Check sheet for the modelled part. Datum: model origin and axes. Units: mm. Give positions to 0.01 mm unless a question says otherwise; leave off trailing zeros. Order: outer loops, then holes, each group sorted by start corner. A loop starts at its lowest first (then second) coordinate and runs counter-clockwise, first axis right, second up.
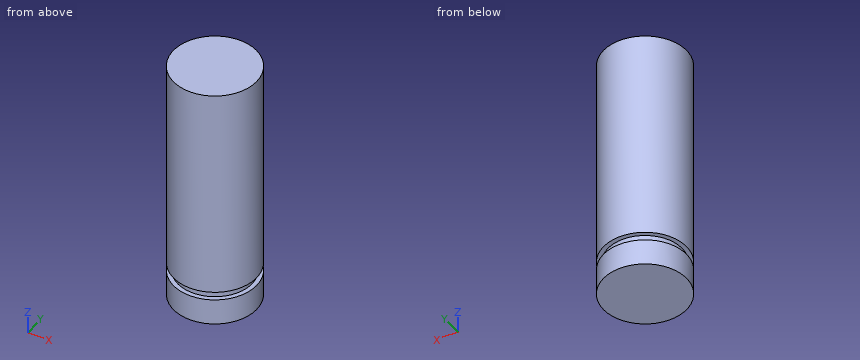
from build123d import *

# Parameters (mm, degrees)
SKETCH1_R           = 3.025
BOSS_EXTRUDE1_DEPTH = 18


with BuildPart() as part:
    # Sketch1 → Boss-Extrude1 (new body)
    with BuildSketch(Plane.XY):
        Circle(SKETCH1_R)
    extrude(amount=BOSS_EXTRUDE1_DEPTH)

    # Sketch3 → Groove for ANSI B27.7 - 3BM1-8, Basic Internal Retaining Ring1 (revolve, cut)
    with BuildSketch(Plane(origin=(0, 0, 18), x_dir=(0, 1, 0), z_dir=(-1, 0, 0)), mode=Mode.PRIVATE) as groove_for_ansi_b27_7_3bm1_8_basic_in_sk:
        with BuildLine():
            Line((4.1, 15.5), (2.7, 15.5))
            Line((2.7, 15.5), (2.7, 16.1))
            Line((2.7, 16.1), (4.1, 16.1))
            ThreePointArc((4.1, 16.1), (4.170710678, 16.070710678), (4.2, 16))
            Line((4.2, 16), (4.2, 15.6))
            ThreePointArc((4.2, 15.6), (4.170710678, 15.529289322), (4.1, 15.5))
        make_face()
    revolve(groove_for_ansi_b27_7_3bm1_8_basic_in_sk.sketch.rotate(Axis((0, 0, 68), (0, 0, -1)), 270), axis=Axis((0, 0, 68), (0, 0, -1)), mode=Mode.SUBTRACT)


solid = part.part
1) Depth check by flat-ended pin: pin 1 Ø1 at (x, z) = (2, 10.5) entering from -Y. Enter the tip coordinate at first touch or a pass-through.
Recorded:
pin 1: stops at y = -2.63
2) Section check B-B, the plane z = 10. Record the cut outline in (x, y) (3 decimals), then the cut area to 3 significant figures.
Recorded:
outline: circle Ø6.05 at (0, 0)
area: 28.7 mm2
3) Section check C-C, the plane y = -1. Record the cut outline in (x, z), then the cut area to 3 significant figures.
Recorded:
outline: (-2.85, 0) - (2.85, 0) - (2.85, 1.9) - (2.51, 1.9) - (2.51, 2.5) - (2.85, 2.5) - (2.85, 18) - (-2.85, 18) - (-2.85, 2.5) - (-2.51, 2.5) - (-2.51, 1.9) - (-2.85, 1.9) - close
area: 102 mm2
4) Material ranges on L1, parallel to Y at x = -0.5, z = 3; L2, parallel to X at y = -1, z = 16.75; L3, parallel to X at y = -2.5, z = 9.5, recorded low to high.
Recorded:
L1: y = -2.98 to 2.98
L2: x = -2.85 to 2.85
L3: x = -1.7 to 1.7
5) Section check A-A, the plane x = 1.5. Record the cut outline in (y, z) (3 decimals), then the cut area to 3 significant figures.
Recorded:
outline: (-2.627, 0) - (2.627, 0) - (2.627, 1.9) - (2.245, 1.9) - (2.245, 2.5) - (2.627, 2.5) - (2.627, 18) - (-2.627, 18) - (-2.627, 2.5) - (-2.245, 2.5) - (-2.245, 1.9) - (-2.627, 1.9) - close
area: 94.1 mm2
